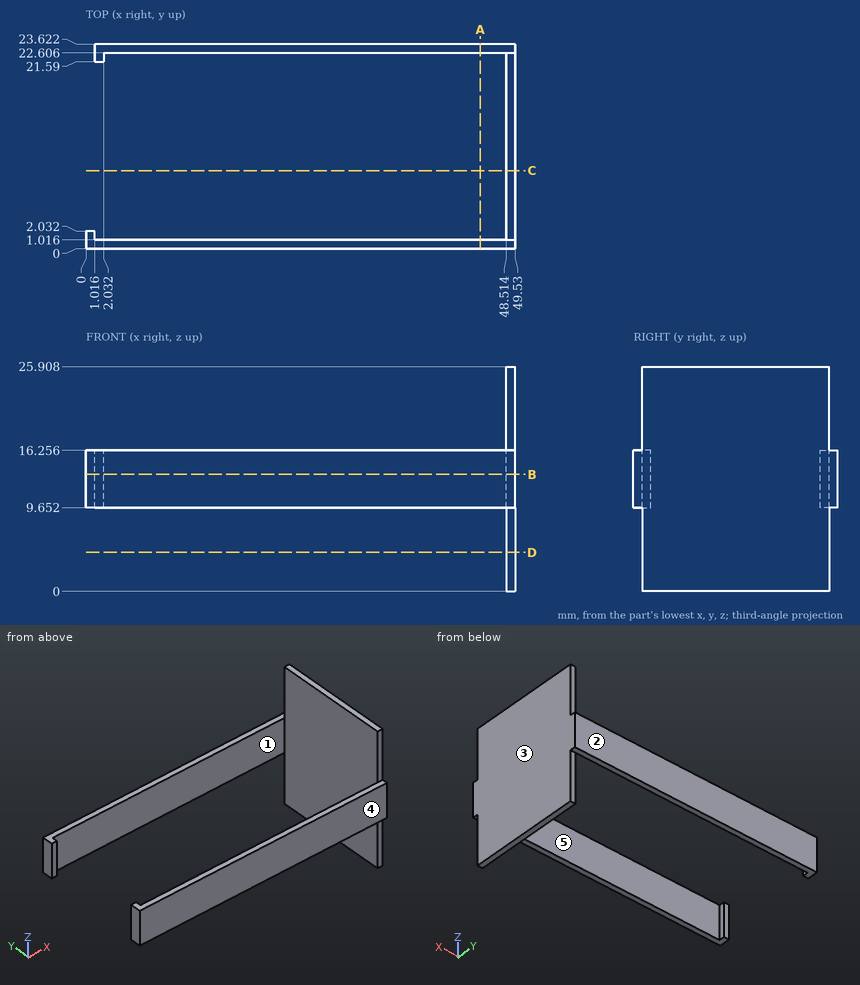
Could you check a few things on this drawing? It's one solid part, dimensions in mm from its lowest x, y, z. A direction names the side the tool comes from. Round coordinates to 2 decimals unless told otherwise and drop trailing zeros. Write each loop counter-clockwise with the first axis right and the second up, starting at its lowest first coordinate (ties: lowest second). Pieces come first, ordered by that corner, then holes.
Q1. If we section it at C-C on y = 9: Write out the boundary of the cut face in (x, z).
Q2. Will these pins go through, and if not, where does the flat tip stop? P1, Ø1, axis at x = 23, y = 22.5, coming from the -Z side; P2, Ø11, axis at y = 6.5, z = 16.5, coming from the -X side; P3, Ø0.5, axis at x = 49, z = 7, coming from the -Y side; P4, Ø0.5, axis at x = 49, z = 5.5, coming from the +Y side.
Q3. If we section it at B-B on z = 13.5: Write out the boundary of the cut face in (x, y).
Q4. Please list where these lines run through material, in increasing order: probe 1 along Y at (x, z) = (38.5, 14); probe 2 along X at (y, z) = (1.25, 23).
Q5. If we section it at A-A on x = 45.5: Write out the boundary of the cut face in (y, z), plus the area to 3 significant figures.
Q6. If we section it at D-D on z = 4.5: Write out the boundary of the cut face in (x, y).
Q7. If we mould it in two halves opening along Y, with no side actions, what happens to the marked faces 3, 4 and 5? For each: +Y half, -Y half, draft (parallel to the pull), parting line (faces both ways), or undercut.
Q8. Which directions (+Z, -Z, +X, -X, +Y, -Y) give clear straight access to the entire face, cutting with the end or side of a thin tool? Please do the marked faces 1 and 2.
Answer below:
1. outline: (48.51, 0) - (49.53, 0) - (49.53, 25.91) - (48.51, 25.91) - close
2. P1: stops at z = 9.65
2. P2: stops at x = 0
2. P3: stops at y = 1.02
2. P4: stops at y = 22.61
3. outline: (0, 0) - (49.53, 0) - (49.53, 23.62) - (1.02, 23.62) - (1.02, 21.59) - (2.03, 21.59) - (2.03, 22.61) - (48.51, 22.61) - (48.51, 1.02) - (1.02, 1.02) - (1.02, 2.03) - (0, 2.03) - close
4. probe 1: y = 0 to 1.02, 22.61 to 23.62
4. probe 2: x = 48.51 to 49.53
5. outline: (0, 9.65) - (1.02, 9.65) - (1.02, 16.26) - (0, 16.26) - close; (22.61, 9.65) - (23.62, 9.65) - (23.62, 16.26) - (22.61, 16.26) - close
5. area: 13.4 mm2
6. outline: (48.51, 1.02) - (49.53, 1.02) - (49.53, 22.61) - (48.51, 22.61) - close
7. face 3: draft
7. face 4: -Y half
7. face 5: undercut
8. face 1: +Z, -Z
8. face 2: +Z, -Z, +X, -X, +Y
